The drawing under review shows one solid part. Ordinate dimensions are in mm from its lowest x, y, z. Give positions to 0.01 mm unless a question says otherwise; leave off trailing zeros. Loops run counter-clockwise (first coordinate to the right, second up) from the corner with the lowest first, then second, coordinate; pieces in that order, holes last. Notation, with made-up numbers: M -23.5,-28 L -19.5,-28 A24 ccw -19.5,11 Z; hole C 78.25,54 d7. An arc over 180 degrees is marked long. Put each result on its own line as item: value. Start each with the question number.
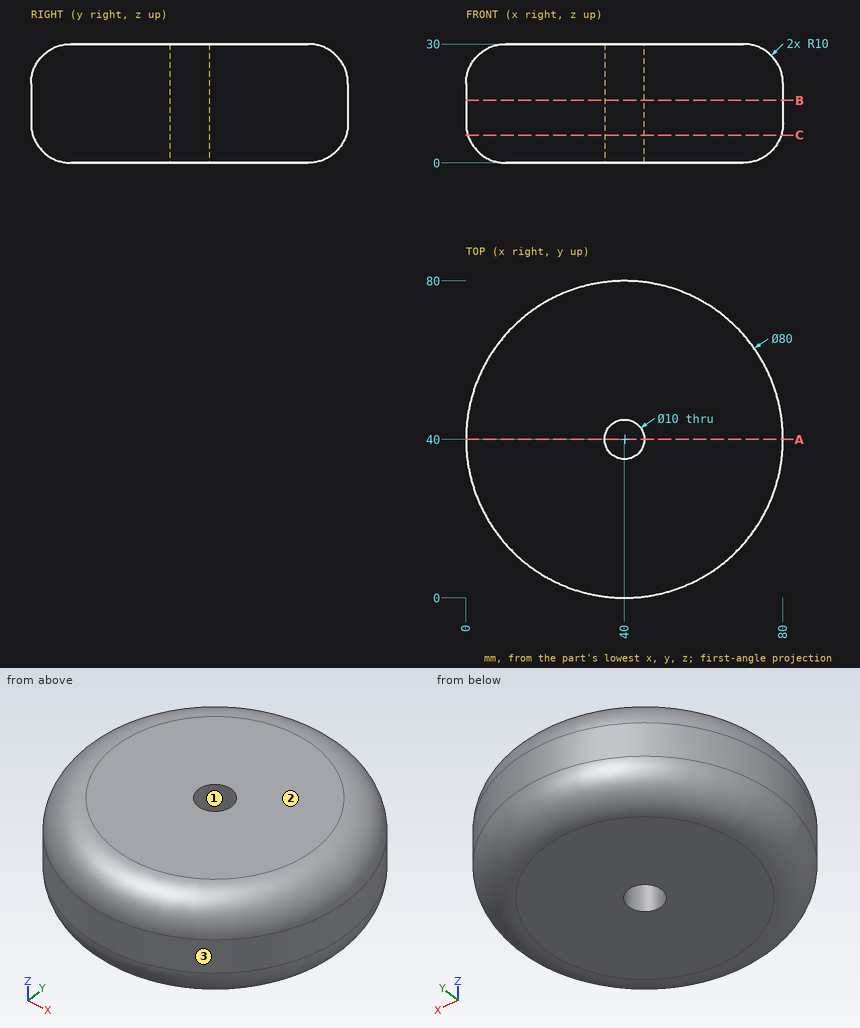
(1) Draft analysis for pull direction X (two halves, no side actions). For the marked faces 1, 2 and 3, state which applies: +X half, -X half, draft (parallel to the pull), parting line (faces both ways), or undercut.
(2) To check wall thickness, follow L1, parallel to Y at x = 40, z = 15; L2, parallel to Y at x = 40, z = 21; L3, parallel to X at y = 37.5, z = 11.75. State the ranges of each line that lie inside material, in increasing order. Write a range as [from, to].
(3) We need section B-B, the plane z = 15.75. Write out the cut boundary in (x, y), plus the area to 3 significant figures.
(4) We need section A-A, the plane y = 40. Write out the cut boundary in (x, z).
(5) Insertion check: pin 1 (4 mm diameter, centred on y = 47, z = 11.5, fed in from -X); pin 2 (3 mm diameter, centred on y = 53.5, z = 21.5, fed in from -X); pin 3 (6 mm diameter, centred on y = 51, z = 13, fed in from -X). Each pin has a flat end and moves straight along its axis. Give the tip position at first contact, or say it passes through.
(6) We need section C-C, the plane z = 7. Write out the cut boundary in (x, y), plus the area to 3 significant figures.
Check sheet entries:
1. face 1: undercut
1. face 2: draft
1. face 3: parting line
2. L1: y = [0, 35], [45, 80]
2. L2: y = [0.05, 35], [45, 79.95]
2. L3: x = [0.08, 35.67], [44.33, 79.92]
3. outline: C 40,40 d80; hole C 40,40 d10
3. area: 4,950 mm²
4. outline: M 0,10 A10 ccw 10,0 L 35,0 L 35,30 L 10,30 A10 ccw 0,20 Z; M 45,0 L 70,0 A10 ccw 80,10 L 80,20 A10 ccw 70,30 L 45,30 Z
5. pin 1: stops at x = 0.31
5. pin 2: stops at x = 1.92
5. pin 3: stops at x = 0.81
6. outline: C 40,40 d79.08; hole C 40,40 d10
6. area: 4,830 mm²
